Model file for the job. Use its own axes, mm. A direction names the side the tool comes from. Give positions to 0.01 mm unless a question says otherwise; leave off trailing zeros. Loops run counter-clockwise (first coordinate to the right, second up) from the corner with the lowest first, then second, coordinate; pieces in that order, holes last. Notation, with made-up numbers: M 80,30.5 L 115,30.5 A22 ccw 115,46.5 Z; hole C -15.5,-10 d4. An arc over 180 degrees is marked long. Answer in a Markdown table with one row per item.
```python
from build123d import *
from OCP.BRepFilletAPI import BRepFilletAPI_MakeFillet

# Parameters (mm, degrees)
SKETCH1_W                         = 37.5
SKETCH1_H                         = 130
MOUNTING_PLATE_DEPTH              = 6.5
M3_CLEARANCE_SLOT1_DEPTH          = 6.5
LPATTERN4_COUNT                   = 2
LPATTERN4_PITCH                   = 31
LPATTERN4_COUNT_DIR2              = 2
LPATTERN4_PITCH_DIR2              = 31
CUT_EXTRUDE3_DEPTH                = 136.456635127
LIMIT_SWITCH_PLACEMENT_DEPTH      = 136.456635127
LIMIT_SWITCH_PLACEMENT_DEPTH_BACK = 136.456635127
M2X0_4_TAPPED_HOLE3_D             = 1.6
LPATTERN5_COUNT                   = 5
LPATTERN5_PITCH                   = 20
FILLET1_R1                        = 5
FILLET1_R2                        = 1
M3X0_5_TAPPED_HOLE1_D             = 2.5
M3X0_5_TAPPED_HOLE1_DEPTH         = 7.5
M3X0_5_TAPPED_HOLE1_TIP           = 0.751075774
LPATTERN3_COUNT                   = 2
LPATTERN3_PITCH                   = 5
LPATTERN6_COUNT                   = 2
LPATTERN6_PITCH                   = 15
LPATTERN6_COUNT_DIR2              = 2
LPATTERN6_PITCH_DIR2              = 20
SKETCH30_R                        = 2.5
CUT_EXTRUDE4_DEPTH                = 136.456635127


# Read off the part's stored shape, not the designer's step: M3 Clearance Slot1
with BuildPart() as part:
    # Sketch1 → Mounting Plate (new body)
    with BuildSketch(Plane.XY):
        with Locations((-18.75, 65)):
            Rectangle(SKETCH1_W, SKETCH1_H)
        with Locations((18.75, 65)):
            Rectangle(SKETCH1_W, SKETCH1_H)
    extrude(amount=MOUNTING_PLATE_DEPTH)

    # M3 Clearance Slot1 outline → M3 Clearance Slot1 (cut)
    with BuildSketch(Plane.XY):
        with BuildLine():
            Line((2.2, 121.7), (2.2, 126.3))
            ThreePointArc((2.2, 126.3), (0.5, 128), (-1.2, 126.3))
            Line((-1.2, 126.3), (-1.2, 121.7))
            ThreePointArc((-1.2, 121.7), (0.5, 120), (2.2, 121.7))
        make_face()
    m3_clearance_slot1 = extrude(amount=M3_CLEARANCE_SLOT1_DEPTH, mode=Mode.SUBTRACT)

    # LPattern4: M3 Clearance Slot1 2 × 2
    with Locations(*[(i * LPATTERN4_PITCH, -j * LPATTERN4_PITCH_DIR2, 0) for i in range(LPATTERN4_COUNT) for j in range(LPATTERN4_COUNT_DIR2) if (i, j) != (0, 0)]):
        add(m3_clearance_slot1, mode=Mode.SUBTRACT)

    # Sketch23 → Cut-Extrude3 (cut, through all)
    with BuildSketch(Plane.XY.offset(6.5)):
        with BuildLine():
            Line((27, 111), (27, 106))
            ThreePointArc((27, 106), (16, 95), (5, 106))
            Line((5, 106), (5, 111))
            ThreePointArc((5, 111), (16, 122), (27, 111))
        make_face()
    extrude(amount=-CUT_EXTRUDE3_DEPTH, mode=Mode.SUBTRACT)

    # Sketch2 → Limit Switch Placement (cut, two sides: drawn at the far end of the back side and taken through both)
    with BuildSketch(Plane.XY.offset(6.5).offset(-LIMIT_SWITCH_PLACEMENT_DEPTH_BACK)):
        with BuildLine():
            Line((-7.5, 415.136329844), (-7.5, 130))
            Line((-7.5, 130), (-7.5, 115))
            ThreePointArc((-7.5, 115), (-10.428932188, 107.928932188), (-17.5, 105))
            Line((-17.5, 105), (-37.5, 105))
            Line((-37.5, 105), (-322.636329844, 105))
            Line((-322.636329844, 105), (-722.642663203, 511.455212366))
            Line((-722.642663203, 511.455212366), (-407.50633336, 821.59154221))
            Line((-407.50633336, 821.59154221), (-7.5, 415.136329844))
        make_face()
    extrude(amount=LIMIT_SWITCH_PLACEMENT_DEPTH + LIMIT_SWITCH_PLACEMENT_DEPTH_BACK, mode=Mode.SUBTRACT)

    # M2x0.4 Tapped Hole3 (through all)
    with Locations(Plane.XY.offset(6.5)):
        with Locations((-17.5, 95)):
            m2x0_4_tapped_hole3 = Hole(M2X0_4_TAPPED_HOLE3_D / 2)

    # LPattern5: M2x0.4 Tapped Hole3 ×5
    with Locations(*[(0, -i * LPATTERN5_PITCH, 0) for i in range(1, LPATTERN5_COUNT)]):
        add(m2x0_4_tapped_hole3, mode=Mode.SUBTRACT)

    # Fillet1: one fillet with a radius per group of edges: ONE call of the kernel's fillet builder (fillet() takes one radius for all edges)
    fillet1_edges_1 = [part.edges().sort_by_distance(p)[0] for p in [
        (37.5, 130, 3.25),
        (37.5, 0, 3.25),
        (-37.5, 0, 3.25),
        (-7.5, 130, 3.25),
    ]]
    fillet1_edges_2 = [part.edges().sort_by_distance(p)[0] for p in [
        (-37.5, 105, 3.25),
    ]]
    fillet1 = BRepFilletAPI_MakeFillet(part.part.solid().wrapped)
    for e in fillet1_edges_1:
        fillet1.Add(FILLET1_R1, e.wrapped)
    for e in fillet1_edges_2:
        fillet1.Add(FILLET1_R2, e.wrapped)
    add(Compound.cast(fillet1.Shape()), mode=Mode.REPLACE)

    # M3x0.5 Tapped Hole1
    with Locations(Plane(origin=(0, 0, 0), x_dir=(-1, 0, 0), z_dir=(0, -1, 0))):
        with Locations((-18.5, -3.25), (-12.5, -3.25)):
            Hole(M3X0_5_TAPPED_HOLE1_D / 2, depth=M3X0_5_TAPPED_HOLE1_DEPTH)
            with Locations((0, 0, -(M3X0_5_TAPPED_HOLE1_DEPTH + M3X0_5_TAPPED_HOLE1_TIP / 2))):  # 118° drill point
                Cone(0, M3X0_5_TAPPED_HOLE1_D / 2, M3X0_5_TAPPED_HOLE1_TIP, mode=Mode.SUBTRACT)

    # Sketch15 → M2x0.4 Tapped Hole2 (revolve, cut)
    with BuildSketch(Plane(origin=(-33.5, 105, 3.25), x_dir=(0, 0, 1), z_dir=(1, 0, 0))):
        Polygon((0, 0), (0, 5.680688495), (0.8, 5.2), (0.8, 0.225), (1.025, 0), align=None)
    m2x0_4_tapped_hole2 = revolve(axis=Axis((-33.5, 111.35, 3.25), (0, -1, 0)), mode=Mode.SUBTRACT)

    # LPattern3: M2x0.4 Tapped Hole2 ×2
    with Locations(*[(i * LPATTERN3_PITCH, 0, 0) for i in range(1, LPATTERN3_COUNT)]):
        add(m2x0_4_tapped_hole2, mode=Mode.SUBTRACT)

    # Sketch29 → M3x0.5 Tapped Hole4 (revolve, cut)
    with BuildSketch(Plane(origin=(23.5, 40, 0), x_dir=(0, 1, 0), z_dir=(1, 0, 0))):
        Polygon((0, 0), (0, 6.251075774), (1.25, 5.5), (1.25, 0), align=None)
    m3x0_5_tapped_hole4 = revolve(axis=Axis((23.5, 40, -6.35), (0, 0, 1)), mode=Mode.SUBTRACT)

    # LPattern6: M3x0.5 Tapped Hole4 2 × 2
    with Locations(*[(-i * LPATTERN6_PITCH, -j * LPATTERN6_PITCH_DIR2, 0) for i in range(LPATTERN6_COUNT) for j in range(LPATTERN6_COUNT_DIR2) if (i, j) != (0, 0)]):
        add(m3x0_5_tapped_hole4, mode=Mode.SUBTRACT)

    # Sketch30 → Cut-Extrude4 (cut, through all)
    with BuildSketch(Plane.XY.offset(6.5)):
        with Locations((15.5, 10)):
            Circle(SKETCH30_R)
    extrude(amount=-CUT_EXTRUDE4_DEPTH, mode=Mode.SUBTRACT)


solid = part.part
```
Q1. Saw through at B-B (x = 0.5). Give the cut face in (y, z).
Reported:
| item | result |
|---|---|
| outline | M 0,0 L 89,0 L 89,6.5 L 0,6.5 Z; M 97,0 L 120,0 L 120,6.5 L 97,6.5 Z; M 128,0 L 130,0 L 130,6.5 L 128,6.5 Z |
Q2. Saw through at C-C (z = 1). Give the number of separate pieces and of enclosed holes in the cut face, and give its area (3 significant figures).
Reported:
| item | result |
|---|---|
| separate pieces | 1 |
| enclosed holes | 15 |
| area | 8,360 mm² |
Q3. Drop flat-ended pins along their axis: pin 1 (2.5 mm diameter, centred on y = 123.5, z = 2.5, fed in from -X); pin 2 (2.5 mm diameter, centred on x = -28.5, z = 3.25, fed in from +Y); pin 3 (3 mm diameter, centred on x = 15.5, y = 10, fed in from +Z); pin 4 (2.5 mm diameter, centred on y = 109.5, z = 2, fed in from -X). Give the stop position or say it passes through.
Reported:
| item | result |
|---|---|
| pin 1 | x = -7.5 |
| pin 2 | y = 105 |
| pin 3 | through |
| pin 4 | x = -10.12 |
Q4. Saw through at D-D (x = -24.5). Give the cut face in (y, z).
Reported:
| item | result |
|---|---|
| outline | M 0,0 L 105,0 L 105,6.5 L 0,6.5 Z |
Q5. 3-axis set-ups, long thin cutter, end or side, ignore diameter. For faces 1 (the face through (19.655, 3.802, 3.729)), 2 (the face through (-7.5, 120, 3)), 3 (the face through (23.43, 20.21, 6.12)), 4 (the face through (31.5, 120, 3.2)): which of +Z, -Z, +X, -X, +Y, -Y reach the whole face in a straight line?
Reported:
| item | result |
|---|---|
| face 1 | -Y |
| face 2 | +Z, -Z, -X, +Y |
| face 3 | -Z |
| face 4 | +Z, -Z |
Q6. Probe probe 1 along Y at (x, z) = (-17.5, 2.5); probe 2 along X at (y, z) = (20, 4.2); probe 3 along X at (y, z) = (75, 3.25). List the from-to ranges inside material, lowest first.
Reported:
| item | result |
|---|---|
| probe 1 | 0 to 14.2, 15.8 to 34.2, 35.8 to 54.2, 55.8 to 74.2, 75.8 to 94.2, 95.8 to 105 |
| probe 2 | -37.5 to 7.25, 9.75 to 22.25, 24.75 to 37.5 |
| probe 3 | -37.5 to -18.3, -16.7 to 37.5 |
Q7. Mould opens along Y. For faces 5 (the face through (-37.5, 54, 3)), 6 (the face through (0.5, 120, 3.2)), 7 (the face through (29.8, 93, 3)), 8 (the face through (18.3, 8.12, 3.33)) say: released by +Y, released by -Y, zero draft, split by the parting line, or undercut.
Reported:
| item | result |
|---|---|
| face 5 | zero draft |
| face 6 | undercut |
| face 7 | undercut |
| face 8 | released by -Y |
Q8. Saw through at A-A (y = 10). Give the cut face in (x, z), and give its area (3 significant figures).
Reported:
| item | result |
|---|---|
| outline | M -37.5,0 L 13,0 L 13,6.5 L -37.5,6.5 Z; M 18,0 L 37.5,0 L 37.5,6.5 L 18,6.5 Z |
| area | 455 mm² |
